from build123d import *

# Parameters (mm, degrees)
SKETCH_1_R          = 7.5
SKETCH_1_R_2        = 3
EXTRUDE_1_DEPTH     = 15
SKETCH_1_3_R        = 10
SKETCH_1_3_R_2      = 7.5
EXTRUDE_2_DEPTH     = 5
SKETCH_2_R          = 1.4
CUT_EXTRUDE_1_DEPTH = 22.5
CHAMFER_1_SIZE      = 1


with BuildPart() as part:
    # 스케치1 → 보스-돌출1 (new body)
    with BuildSketch(Plane.XY):
        Circle(SKETCH_1_R)
        Circle(SKETCH_1_R_2, mode=Mode.SUBTRACT)
    extrude(amount=EXTRUDE_1_DEPTH)

    # 스케치1<3> → 보스-돌출2 (add)
    with BuildSketch(Plane.XY):
        Circle(SKETCH_1_3_R)
        Circle(SKETCH_1_3_R_2, mode=Mode.SUBTRACT)
    extrude(amount=EXTRUDE_2_DEPTH)

    # 스케치2 → 컷-돌출1 (cut, symmetric)
    with BuildSketch(Plane(origin=(0, 0, 0), x_dir=(0, 0, -1), z_dir=(1, 0, 0))):
        with Locations((-10, 0)):
            Circle(SKETCH_2_R)
    extrude(amount=CUT_EXTRUDE_1_DEPTH, both=True, mode=Mode.SUBTRACT)

    # 모따기1
    chamfer_1_edges = [part.edges().sort_by_distance(p)[0] for p in [
        (-3, 0, 0),
        (-3, 0, 15),
    ]]
    chamfer(chamfer_1_edges, length=CHAMFER_1_SIZE)


solid = part.part
Input: part model. Units: mm. Frame: model coordinates. A direction names the side the tool comes from. Give positions to 0.01 mm unless a question says otherwise; leave off trailing zeros. Order: outer loops, then holes, each group sorted by start corner. A loop starts at its lowest first (then second) coordinate and runs counter-clockwise, first axis right, second up. Notation, with made-up numbers: (-2.5, 29.25) - (13.5, 29.25) arc R37 ccw to (13.5, 66.25) - close; hole circle Ø2 at (71.25, -25.5). An arc over 180 degrees is marked (long way). Write each question's results on one line, items separated by ' | '.
Item 1: Section A-A (y = 0). Return loops of the section in (x, z), and give its area (3 significant figures).
A:
outline: (-10, 0) - (-4, 0) - (-3, 1) - (-3, 8.6) - (-7.5, 8.6) - (-7.5, 5) - (-10, 5) - close; (-7.5, 11.4) - (-3, 11.4) - (-3, 14) - (-4, 15) - (-7.5, 15) - close; (3, 1) - (4, 0) - (10, 0) - (10, 5) - (7.5, 5) - (7.5, 8.6) - (3, 8.6) - close; (3, 11.4) - (7.5, 11.4) - (7.5, 15) - (4, 15) - (3, 14) - close | area: 133 mm^2
Item 2: Section B-B (z = 10). Return loops of the section in (x, y), and give its area (3 significant figures).
A:
outline: (-7.37, -1.4) arc R7.5 ccw to (7.37, -1.4) - (2.65, -1.4) arc R3 cw to (-2.65, -1.4) - close; (-7.37, 1.4) - (-2.65, 1.4) arc R3 cw to (2.65, 1.4) - (7.37, 1.4) arc R7.5 ccw to start | area: 123 mm^2
Item 3: Section D-D (z = 6). Return loops of the section in (x, y).
A:
outline: circle Ø15 at (0, 0); hole circle Ø6 at (0, 0)
Item 4: Draft query along X for faces 3 (the cylindrical face through (-5.04, 0.06, 11.4)), 4 (the cylindrical face through (2.86, 0.9, 7.41)), 5 (the cylindrical face through (6.93, -2.87, 9.93)). Return one class per face: released by +X, released by -X, zero draft, split by the parting line, or undercut.
A:
face 3: zero draft | face 4: undercut | face 5: split by the parting line
Item 5: Section C-C (x = 0). Return loops of the section in (y, z).
A:
outline: (-10, 0) - (-4, 0) - (-3, 1) - (-3, 14) - (-4, 15) - (-7.5, 15) - (-7.5, 5) - (-10, 5) - close; (3, 1) - (4, 0) - (10, 0) - (10, 5) - (7.5, 5) - (7.5, 15) - (4, 15) - (3, 14) - close
Item 6: Contact query for flat-ended pins moving along their axis: pin 1 Ø3.5 at (y, z) = (0, 10) entering from -X; pin 2 Ø8 at (x, z) = (6, 1.5) entering from -Y; pin 3 Ø2 at (x, z) = (-1.5, 12) entering from -Y; pin 4 Ø10 at (x, y) = (0, 0.5) entering from +Z. Output: stop coordinate, or through.
A:
pin 1: stops at x = -7.5 | pin 2: stops at y = -9.8 | pin 3: stops at y = -7.48 | pin 4: stops at z = 15
Item 7: Access query for faces 1 (the flat face through (4, 7, 5)), 2 (the flat face through (3, -3, 15)). Directions: +Z, -Z, +X, -X, +Y, -Y. A direction counts if a zero-diameter tool reaches every point of the face in a straight line with its end or side. Return the directions, or none.
A:
face 1: +Z | face 2: +Z, +X, -X, +Y, -Y
Item 8: Material intervals for line 1 along Z through (x, y) = (5.3, 0); line 2 along X through (y, z) = (0, 6); line 3 along Z through (x, y) = (7.75, 1.5), sorted ascending.
A:
line 1: z = 0 to 8.6, 11.4 to 15 | line 2: x = -7.5 to -3, 3 to 7.5 | line 3: z = 0 to 5
